from build123d import *

# Parameters (mm, degrees)
F0_W     = 152.4
F0_H     = 101.6
F1_DEPTH = 127
F2_W     = 63.5
F2_H     = 50.8
F3_DEPTH = 103.87561
F4_R     = 23.014018
F6_DEPTH = 152.401


with BuildPart() as f1:
    # F0 (on Top) → F1 (new body)
    with BuildSketch(Plane.XY):
        with Locations((27.437925, 9.498095)):
            Rectangle(F0_W, F0_H)
    extrude(amount=F1_DEPTH)

    # F2 (on face) → F3 (cut)
    with BuildSketch(Plane.XZ.offset(41.301905)):
        with Locations((71.887925, 101.6)):
            Rectangle(F2_W, F2_H)
    extrude(amount=-F3_DEPTH, mode=Mode.SUBTRACT)

    # F4 (on face) → F6 (cut, through all)
    with BuildSketch(Plane(origin=(-48.762075, 0, 0), x_dir=(0, -1, 0), z_dir=(-1, 0, 0))):
        with Locations((-9.498095, 38.1)):
            Circle(F4_R)
    extrude(amount=-F6_DEPTH, mode=Mode.SUBTRACT)


solid = f1.part
The model under review builds one solid part; all positions refer to its coordinate system, in mm. A direction names the side the tool comes from. Give positions to 0.01 mm unless a question says otherwise; leave off trailing zeros. Write each loop counter-clockwise with the first axis right and the second up, starting at its lowest first coordinate (ties: lowest second). Pieces come first, ordered by that corner, then holes.
1. Add section B-B, the plane y = 5. Write out the cut boundary in (x, z), plus the area to 3 significant figures.
2. For P1, Ø19, axis at x = 68, y = 1.5, coming from the +Z side, flat-tipped, find the tip position at first contact; note if it passes through.
3. Draft analysis for pull direction Y (two halves, no side actions). For faces 1 (the flat face through (26, 10, 0)), 2 (the flat face through (9, -41.302, 48)), 3 (the cylindrical face through (26.371, 14.487, 15.633)), 4 (the flat face through (9, 60.298, 48)), state which applies: +Y half, -Y half, draft (parallel to the pull), parting line (faces both ways), or undercut.
4. Add section C-C, the plane x = 61.5. Write out the cut boundary in (y, z).
5. Wall thickness on L1, parallel to Z at x = -34.5, y = 9; L2, parallel to Z at x = 65, y = -17; L3, parallel to Z at x = 93, y = -9: over which ranges is each line inside the solid? List them lowest first.
6. Add section D-D, the plane y = -6. Write out the cut boundary in (x, z).
7. Tool access review of faces 5 (the flat face through (71, 9, 76.2)), 6 (the flat face through (-48.762, 9, 63)): name each direction out of +Z, -Z, +X, -X, +Y, -Y from which nothing blocks a thin tool from reaching the whole face with its end or side.
8. Add section A-A, the plane z = 38.1. Write out the cut boundary in (x, y), plus the area to 3 significant figures.
Worked answers:
1. outline: (-48.76, 0) - (103.64, 0) - (103.64, 15.53) - (-48.76, 15.53) - close; (-48.76, 60.67) - (103.64, 60.67) - (103.64, 76.2) - (40.14, 76.2) - (40.14, 127) - (-48.76, 127) - close
1. area: 9,250 mm2
2. P1: stops at z = 76.2
3. face 1: draft
3. face 2: -Y half
3. face 3: undercut
3. face 4: +Y half
4. outline: (-41.3, 0) - (60.3, 0) - (60.3, 76.2) - (-41.3, 76.2) - close; hole circle Ø46.03 at (9.5, 38.1)
5. L1: z = 0 to 15.09, 61.11 to 127
5. L2: z = 0 to 76.2
5. L3: z = 0 to 24.41, 51.79 to 76.2
6. outline: (-48.76, 0) - (103.64, 0) - (103.64, 21.09) - (-48.76, 21.09) - close; (-48.76, 55.11) - (103.64, 55.11) - (103.64, 76.2) - (40.14, 76.2) - (40.14, 127) - (-48.76, 127) - close
7. face 5: +Z, +X, +Y, -Y
7. face 6: +Z, -Z, -X, +Y, -Y
8. outline: (-48.76, -41.3) - (103.64, -41.3) - (103.64, -13.52) - (-48.76, -13.52) - close; (-48.76, 32.51) - (103.64, 32.51) - (103.64, 60.3) - (-48.76, 60.3) - close
8. area: 8,470 mm2
